Part model, mm, in its own coordinate system. Face numbers are marked on the shaded views. A direction names the side the tool comes from. Round coordinates to 2 decimals unless told otherwise and drop trailing zeros. Loops run counter-clockwise (first coordinate to the right, second up) from the corner with the lowest first, then second, coordinate; pieces in that order, holes last. Notation, with made-up numbers: (43.25, 74.25) -> (64.25, 74.25) arc R25 cw to (64.25, 108.25) -> close; hole circle Ø1 at (78.25, 16). An arc over 180 degrees is marked (long way). Use a Markdown table: item, result. Add a question column.
Item 1: Flat gauge pins, fed straight in: pin 1 (2 mm diameter, centred on y = 11.5, z = 21, fed in from +X); pin 2 (2 mm diameter, centred on y = 11.5, z = 22, fed in from -X); pin 3 (5 mm diameter, centred on x = 7, z = 3, fed in from +Y). Where does each tip first touch, or does it go through?
Item 2: Probe line 1 (Z direction, x = 7, y = -15.8); line 2 (X direction, y = 0, z = 13.05); line 3 (Z direction, x = -3.5, y = -11). List the from-to ranges inside material, lowest first. Write a range as [from, to].
Item 3: Cut at A-A, the plane z = 14. List the corners of the cut face in (x, y).
Item 4: Which spindle directions (+Z, -Z, +X, -X, +Y, -Y) get a long thin tool onto all of the face, cutting with end or side? Do the marked faces 1, 2 and 3. Say none if no direction does.
Item 5: Two-plate mould, pull along Y, no slides. Class the marked faces 4, 5 and 6: pulls with the +Y half, pulls with the -Y half, needs draft (parallel to the pull), parting line crosses it, or undercut.
Item 6: Cut at B-B, the plane y = 0. List the corners of the cut face in (x, z).
Item 7: Cut at D-D, the plane z = 3. List the corners of the cut face in (x, y).
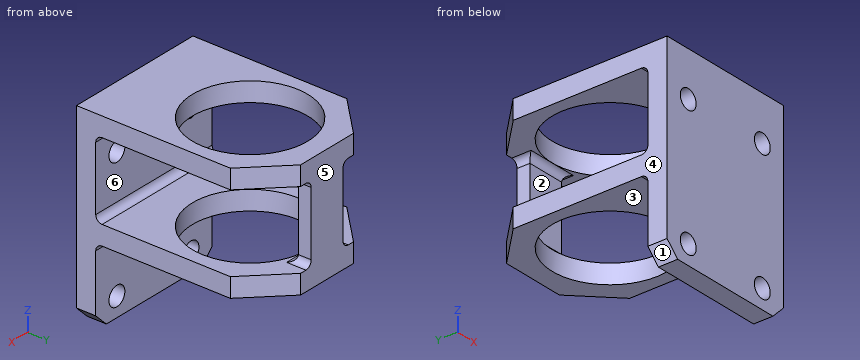
```python
from build123d import *

# Parameters (mm, degrees)
SKETCH_1_W          = 22
SKETCH_1_H          = 30
SKETCH_1_R          = 9
EXTRUDE_2_DEPTH     = 30
SKETCH_4_W          = 12
SKETCH_4_H          = 25
SKETCH_4_H_2        = 30
CUT_EXTRUDE_3_DEPTH = 42.32795664
CHAMFER_2_SIZE      = 2
CUT_EXTRUDE_4_REACH = 45.829
SKETCH_6_R          = 1.5
CUT_EXTRUDE_5_DEPTH = 42.833001327
CHAMFER_3_SIZE      = 6
FILLET_1_R          = 1


with BuildPart() as part:
    # Sketch 1 → Extrude 2 (new body)
    with BuildSketch(Plane.XY):
        with Locations((0, -3)):
            Rectangle(SKETCH_1_W, SKETCH_1_H)
        Circle(SKETCH_1_R, mode=Mode.SUBTRACT)
    extrude(amount=EXTRUDE_2_DEPTH)

    # Sketch 4 → Cut-Extrude 3 (cut, through all)
    with BuildSketch(Plane(origin=(11, 0, 0), x_dir=(0, 0, -1), z_dir=(1, 0, 0))):
        with Locations((-21, -2.5)):
            Rectangle(SKETCH_4_W, SKETCH_4_H)
        with Locations((-6, 0)):
            Rectangle(SKETCH_4_W, SKETCH_4_H_2)
    extrude(amount=-CUT_EXTRUDE_3_DEPTH, mode=Mode.SUBTRACT)

    # Chamfer 2
    chamfer_2_edges = [part.edges().sort_by_distance(p)[0] for p in [
        (-11, -16.5, 0),
        (11, -16.5, 0),
    ]]
    chamfer(chamfer_2_edges, length=CHAMFER_2_SIZE)

    # Sketch 5 → Cut-Extrude 4 (cut, up to next)
    with BuildSketch(Plane(origin=(0, 12, 0), x_dir=(1, 0, 0), z_dir=(0, 1, 0)), mode=Mode.PRIVATE) as cut_extrude_4_sk1:
        with BuildLine():
            Line((3, -27), (9, -27))
            ThreePointArc((9, -27), (4.757359313, -25.242640687), (3, -21))
            Line((3, -21), (3, -27))
        make_face()
    cut_extrude_4_tool1 = extrude(cut_extrude_4_sk1.sketch, amount=-CUT_EXTRUDE_4_REACH, mode=Mode.PRIVATE) & part.part
    # Sketch 5 → Cut-Extrude 4 (cut, up to next)
    with BuildSketch(Plane(origin=(0, 12, 0), x_dir=(1, 0, 0), z_dir=(0, 1, 0)), mode=Mode.PRIVATE) as cut_extrude_4_sk2:
        with BuildLine():
            Line((9, -27), (11, -27))
            Line((11, -27), (11, -15))
            Line((11, -15), (9, -15))
            ThreePointArc((9, -15), (4.757359313, -16.757359313), (3, -21))
            ThreePointArc((3, -21), (4.757359313, -25.242640687), (9, -27))
        make_face()
    cut_extrude_4_tool2 = extrude(cut_extrude_4_sk2.sketch, amount=-CUT_EXTRUDE_4_REACH, mode=Mode.PRIVATE) & part.part
    # Sketch 5 → Cut-Extrude 4 (cut, up to next)
    with BuildSketch(Plane(origin=(0, 12, 0), x_dir=(1, 0, 0), z_dir=(0, 1, 0)), mode=Mode.PRIVATE) as cut_extrude_4_sk3:
        with BuildLine():
            Line((3, -15), (3, -21))
            ThreePointArc((3, -21), (4.757359313, -16.757359313), (9, -15))
            Line((9, -15), (3, -15))
        make_face()
    cut_extrude_4_tool3 = extrude(cut_extrude_4_sk3.sketch, amount=-CUT_EXTRUDE_4_REACH, mode=Mode.PRIVATE) & part.part
    cut_extrude_4_1 = cut_extrude_4_tool1.solids().sort_by_distance((4.340208, 12, 25.659792))[0]
    add(cut_extrude_4_1, mode=Mode.SUBTRACT)
    cut_extrude_4_2 = cut_extrude_4_tool2.solids().sort_by_distance((7.510217, 12, 21))[0]
    add(cut_extrude_4_2, mode=Mode.SUBTRACT)
    cut_extrude_4_3 = cut_extrude_4_tool3.solids().sort_by_distance((4.340208, 12, 16.340208))[0]
    add(cut_extrude_4_3, mode=Mode.SUBTRACT)
    cut_extrude_4 = cut_extrude_4_1 + cut_extrude_4_2 + cut_extrude_4_3  # Cut-Extrude 4 as one shape, for the pattern or mirror that repeats it

    # Mirror 1: Cut-Extrude 4 across plane
    add(cut_extrude_4.mirror(Plane(origin=(0, 0, 0), x_dir=(0, 0, 1), z_dir=(1, 0, 0))), mode=Mode.SUBTRACT)

    # Sketch 6 → Cut-Extrude 5 (cut, through all)
    with BuildSketch(Plane(origin=(0, -15, 0), x_dir=(1, 0, 0), z_dir=(0, 1, 0))):
        with Locations(Location((7, -23, 0), (0, 0, 180))):
            Circle(SKETCH_6_R)
        with Locations(Location((7, -3, 0), (0, 0, 180))):
            Circle(SKETCH_6_R)
        with Locations((-7, -3)):
            Circle(SKETCH_6_R)
        with Locations((-7, -23)):
            Circle(SKETCH_6_R)
    extrude(amount=-CUT_EXTRUDE_5_DEPTH, mode=Mode.SUBTRACT)

    # Chamfer 3
    chamfer_3_edges = [part.edges().sort_by_distance(p)[0] for p in [
        (11, 12, 13.5),
        (-11, 12, 28.5),
        (11, 12, 28.5),
        (-11, 12, 13.5),
    ]]
    chamfer(chamfer_3_edges, length=CHAMFER_3_SIZE)

    # Fillet 1
    fillet_1_edges = [part.edges().sort_by_distance(p)[0] for p in [
        (0, -15, 27),
        (0, -15, 15),
        (0, -15, 12),
        (3, 11, 27),
        (3, 11, 15),
        (0, 10, 15),
        (0, 10, 27),
        (-3, 11, 27),
        (-3, 11, 15),
    ]]
    fillet(fillet_1_edges, radius=FILLET_1_R - 0.0001)  # a hair under: the kernel refuses the full size


solid = part.part
```
A:
| question | item | result |
|---|---|---|
| 1 | pin 1 | stops at x = 3 |
| 1 | pin 2 | stops at x = -3 |
| 1 | pin 3 | stops at y = -15 |
| 2 | line 1 | z = [0, 1.5], [4.5, 21.5], [24.5, 30] |
| 2 | line 2 | x = [-11, -9], [9, 11] |
| 2 | line 3 | z = [12, 15], [27, 30] |
| 3 | outline | (-11, -18) -> (11, -18) -> (11, 6) -> (5, 12) -> (-5, 12) -> (-11, 6) -> close; hole circle Ø18 at (0, 0) |
| 4 | face 1 | -Z, -X, +Y, -Y |
| 4 | face 2 | +X, -X |
| 4 | face 3 | -Z, +X, -X, +Y |
| 5 | face 4 | needs draft |
| 5 | face 5 | pulls with the +Y half |
| 5 | face 6 | undercut |
| 6 | outline | (-11, 12) -> (-9, 12) -> (-9, 15) -> (-11, 15) -> close; (-11, 27) -> (-9, 27) -> (-9, 30) -> (-11, 30) -> close; (9, 12) -> (11, 12) -> (11, 15) -> (9, 15) -> close; (9, 27) -> (11, 27) -> (11, 30) -> (9, 30) -> close |
| 7 | outline | (-11, -18) -> (-8.5, -18) -> (-8.5, -15) -> (-11, -15) -> close; (-5.5, -18) -> (5.5, -18) -> (5.5, -15) -> (-5.5, -15) -> close; (8.5, -18) -> (11, -18) -> (11, -15) -> (8.5, -15) -> close |
